Study the drawing (mm; zero at the part's minimum x, y, z) and answer. A direction names the side the tool comes from. Round coordinates to 2 decimals unless told otherwise and drop trailing zeros. Write each loop counter-clockwise with the first axis right and the second up, starting at its lowest first coordinate (ties: lowest second). Pieces come first, ordered by that corner, then holes. Notation, with made-up numbers: (64, 32.25) - (106, 32.25) arc R21 cw to (106, 67.25) - close; hole circle Ø4 at (-32.75, 54). An arc over 180 degrees is marked (long way). Return JSON: item names as keys, results as strings. Group by question number.
(1) Section C-C, the plane y = 191 is taken. Write down the section's boundary in (x, z) (1 decimal).
(2) Which of the six approach directions +Z, -Z, +X, -X, +Y, -Y give full straight-line access (tool end or side, diameter ignored) to the marked faces 1, 2 and 3?
(3) Each of these flat-tipped pins is pushed along its axis until it touches: pin 1 (6.5 mm diameter, centred on x = 8.5, z = 34, fed in from +Y); pin 2 (5 mm diameter, centred on x = 61, z = 50.5, fed in from -Y); pin 3 (12 mm diameter, centred on x = 19.5, z = 98.5, fed in from +Y); pin 4 (4 mm diameter, centred on x = 43.5, y = 34.5, fed in from +Z). Where does it stop, or does it pass through?
(4) Section D-D, the plane z = 69.5 is taken. Write down the section's boundary in (x, y).
(5) Find the intervals of material crossed by line 1 along Z through (x, y) = (50, 70) (1 decimal); line 2 along Y through (x, z) = (11, 16); line 3 along X through (y, z) = (11, 47.5), in increasing order. Write a range as [from, to].
(6) Section A-A, the plane z = 53 is taken. Write down the section's boundary in (x, y).
(7) Determine the mould class of the marked faces 4, 5, 6 and 7 for opening direction Y: +Y half, -Y half, draft (parallel to the pull), parting line (faces both ways), or undercut.
(8) Section B-B, the plane x = 39 is taken. Write down the section's boundary in (y, z) (1 decimal).
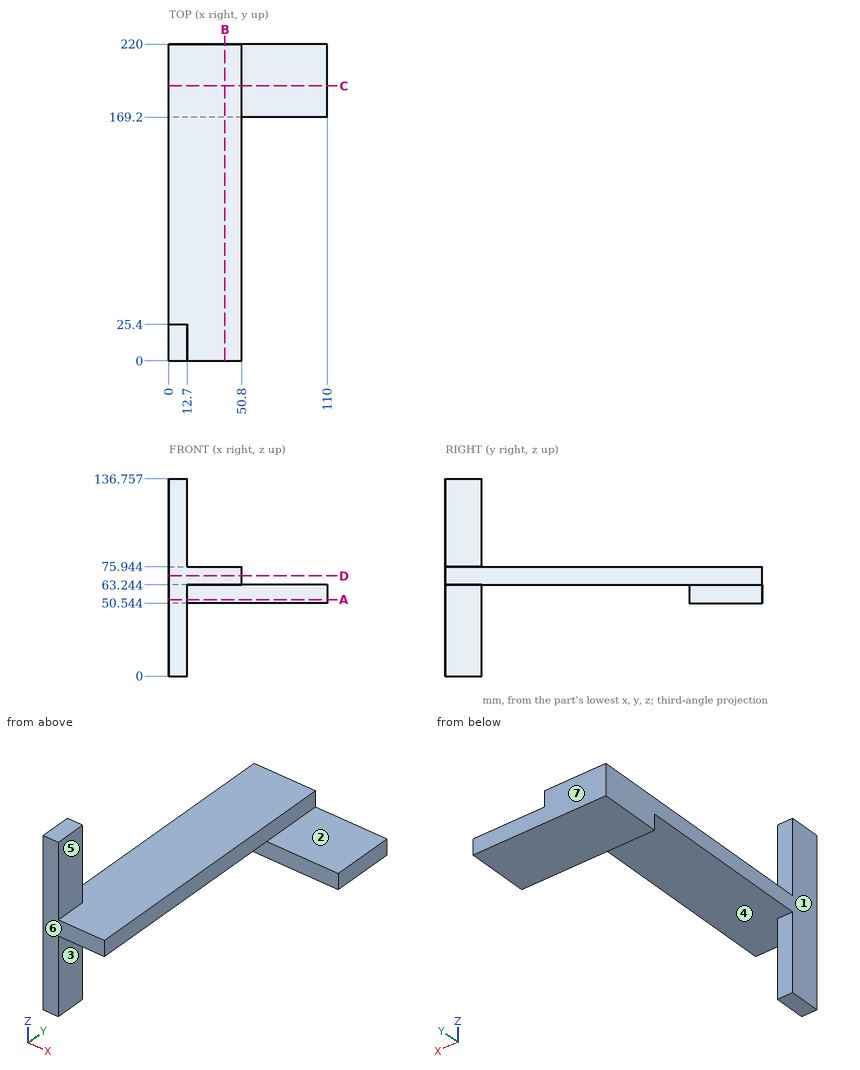
Working result:
{
 "1": {"outline": "(0, 50.5) - (110, 50.5) - (110, 63.2) - (50.8, 63.2) - (50.8, 75.9) - (0, 75.9) - close"},
 "2": {"face 1": "+Z, -Z, -X, +Y, -Y", "face 2": "+Z, +X, +Y, -Y", "face 3": "-Z, +X, -Y"},
 "3": {"pin 1": "stops at y = 25.4", "pin 2": "stops at y = 169.2", "pin 3": "passes through", "pin 4": "stops at z = 75.94"},
 "4": {"outline": "(0, 0) - (50.8, 0) - (50.8, 220) - (0, 220) - close"},
 "5": {"line 1": "z = [63.2, 75.9]", "line 2": "y = [0, 25.4]", "line 3": "x = [0, 12.7]"},
 "6": {"outline": "(0, 0) - (12.7, 0) - (12.7, 25.4) - (0, 25.4) - close; (0, 169.2) - (110, 169.2) - (110, 220) - (0, 220) - close"},
 "7": {"face 4": "undercut", "face 5": "draft", "face 6": "-Y half", "face 7": "+Y half"},
 "8": {"outline": "(0, 63.2) - (169.2, 63.2) - (169.2, 50.5) - (220, 50.5) - (220, 75.9) - (0, 75.9) - close"}
}
